Could you check a few things on this model? Use its own coordinates, in mm. Face numbers are marked on the shaded views. A direction names the side the tool comes from. Round coordinates to 2 decimals unless told otherwise and drop trailing zeros. Loops run counter-clockwise (first coordinate to the right, second up) from the corner with the lowest first, then second, coordinate; pieces in that order, holes last. Notation, with made-up numbers: (72.25, 84) -> (108.25, 84) arc R23 ccw to (108.25, 105) -> close; hole circle Ø10 at (64.25, 82). An arc over 180 degrees is marked (long way). One line per item, written item: value.
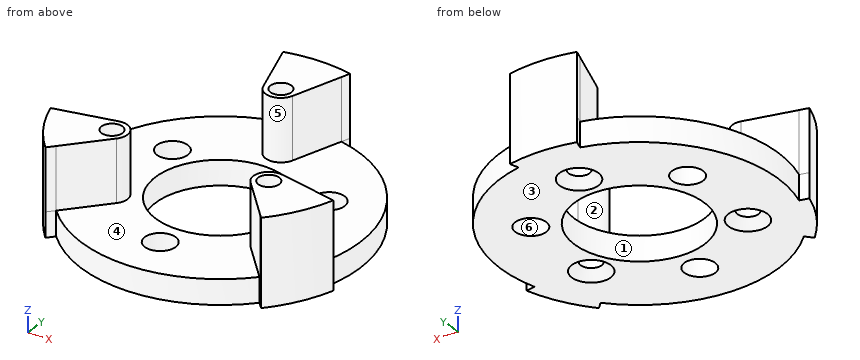
```python
from build123d import *

# Parameters (mm, degrees)
SKETCH1_R                                       = 22.5
SKETCH1_R_2                                     = 10.5
SKETCH1_R_3                                     = 1.5
BOSS_EXTRUDE1_DEPTH                             = 4
BOSS_EXTRUDE4_START                             = -4
SKETCH4_R                                       = 2.5
SKETCH4_R_2                                     = 1.5
BOSS_EXTRUDE4_DEPTH                             = 4
SKETCH4_5_R                                     = 1.5
BOSS_EXTRUDE5_DEPTH                             = 10
CUT_EXTRUDE1_DEPTH                              = 35.690393407
CUT_EXTRUDE1_DEPTH_BACK                         = 35.690393407
SKETCH4_3_R                                     = 2.5
CSK_FOR_M3_FLAT_HEAD_MACHINE_SCREW1_D           = 3.4
CSK_FOR_M3_FLAT_HEAD_MACHINE_SCREW1_CSINK_D     = 6.3
CSK_FOR_M3_FLAT_HEAD_MACHINE_SCREW1_CSINK_ANGLE = 90


with BuildPart() as part:
    # Sketch1 → Boss-Extrude1 (new body)
    with BuildSketch(Plane.XY):
        Circle(SKETCH1_R)
        Circle(SKETCH1_R_2, mode=Mode.SUBTRACT)
        with Locations((12.730573436, -7.35)):
            Circle(SKETCH1_R_3, mode=Mode.SUBTRACT)
        with Locations((0, 14.7)):
            Circle(SKETCH1_R_3, mode=Mode.SUBTRACT)
        with Locations((-12.730573436, -7.35)):
            Circle(SKETCH1_R_3, mode=Mode.SUBTRACT)
    extrude(amount=BOSS_EXTRUDE1_DEPTH)

    # Sketch4 → Boss-Extrude4 (add)
    # profile 1 of 6: a face of its own
    with BuildSketch(Plane.XY.offset(4).offset(BOSS_EXTRUDE4_START)):
        with Locations((0, -14.7)):
            Circle(SKETCH4_R)
    # profile 2 of 6: a face of its own
    with BuildSketch(Plane.XY.offset(4).offset(BOSS_EXTRUDE4_START)):
        with Locations((-12.730573436, 7.35)):
            Circle(SKETCH4_R)
    # profile 3 of 6: a face of its own
    with BuildSketch(Plane.XY.offset(4).offset(BOSS_EXTRUDE4_START)):
        with Locations((12.730573436, 7.35)):
            Circle(SKETCH4_R)
    # profile 4 of 6: a face of its own
    with BuildSketch(Plane.XY.offset(4).offset(BOSS_EXTRUDE4_START)):
        with BuildLine():
            Line((-10.872711372, -9.022826516), (-17.518780447, -16.404034005))
            ThreePointArc((-17.518780447, -16.404034005), (-20.784609691, -12), (-22.965700397, -6.969691908))
            Line((-22.965700397, -6.969691908), (-13.250352663, -4.904630998))
            ThreePointArc((-13.250352663, -4.904630998), (-10.565509926, -6.1), (-10.872711372, -9.022826516))
        make_face()
        with Locations((-12.730573436, -7.35)):
            Circle(SKETCH4_R_2, mode=Mode.SUBTRACT)
    # profile 5 of 6: a face of its own
    with BuildSketch(Plane.XY.offset(4).offset(BOSS_EXTRUDE4_START)):
        with BuildLine():
            Line((2.377641291, 13.927457514), (5.44691995, 23.373725913))
            ThreePointArc((5.44691995, 23.373725913), (0, 24), (-5.44691995, 23.373725913))
            Line((-5.44691995, 23.373725913), (-2.377641291, 13.927457514))
            ThreePointArc((-2.377641291, 13.927457514), (0, 12.2), (2.377641291, 13.927457514))
        make_face()
        with Locations((0, 14.7)):
            Circle(SKETCH4_R_2, mode=Mode.SUBTRACT)
    # profile 6 of 6: a face of its own
    with BuildSketch(Plane.XY.offset(4).offset(BOSS_EXTRUDE4_START)):
        with BuildLine():
            Line((10.872711372, -9.022826516), (17.518780447, -16.404034005))
            ThreePointArc((17.518780447, -16.404034005), (20.784609691, -12), (22.965700397, -6.969691908))
            Line((22.965700397, -6.969691908), (13.250352663, -4.904630998))
            ThreePointArc((13.250352663, -4.904630998), (10.565509926, -6.1), (10.872711372, -9.022826516))
        make_face()
        with Locations((12.730573436, -7.35)):
            Circle(SKETCH4_R_2, mode=Mode.SUBTRACT)
    extrude(amount=BOSS_EXTRUDE4_DEPTH)

    # Sketch4<5> → Boss-Extrude5 (add)
    # profile 1 of 6: a face of its own
    with BuildSketch(Plane.XY.offset(4)):
        with BuildLine():
            Line((-5.44691995, 23.373725913), (-4.981593415, 21.941598097))
            ThreePointArc((-4.981593415, 21.941598097), (0, 22.5), (4.981593415, 21.941598097))
            Line((4.981593415, 21.941598097), (5.44691995, 23.373725913))
            ThreePointArc((5.44691995, 23.373725913), (0, 24), (-5.44691995, 23.373725913))
        make_face()
    # profile 2 of 6: a face of its own
    with BuildSketch(Plane.XY.offset(4)):
        with BuildLine():
            ThreePointArc((4.981593415, 21.941598097), (0, 22.5), (-4.981593415, 21.941598097))
            Line((-4.981593415, 21.941598097), (-2.377641291, 13.927457514))
            ThreePointArc((-2.377641291, 13.927457514), (0, 12.2), (2.377641291, 13.927457514))
            Line((2.377641291, 13.927457514), (4.981593415, 21.941598097))
        make_face()
        with Locations((0, 14.7)):
            Circle(SKETCH4_5_R, mode=Mode.SUBTRACT)
    # profile 3 of 6: a face of its own
    with BuildSketch(Plane.XY.offset(4)):
        with BuildLine():
            Line((-17.518780447, -16.404034005), (-16.511184644, -15.284985497))
            ThreePointArc((-16.511184644, -15.284985497), (-19.485571585, -11.25), (-21.492778059, -6.6566126))
            Line((-21.492778059, -6.6566126), (-22.965700397, -6.969691908))
            ThreePointArc((-22.965700397, -6.969691908), (-20.784609691, -12), (-17.518780447, -16.404034005))
        make_face()
    # profile 4 of 6: a face of its own
    with BuildSketch(Plane.XY.offset(4)):
        with BuildLine():
            Line((-16.511184644, -15.284985497), (-10.872711372, -9.022826516))
            ThreePointArc((-10.872711372, -9.022826516), (-10.565509926, -6.1), (-13.250352663, -4.904630998))
            Line((-13.250352663, -4.904630998), (-21.492778059, -6.6566126))
            ThreePointArc((-21.492778059, -6.6566126), (-19.485571585, -11.25), (-16.511184644, -15.284985497))
        make_face()
        with Locations((-12.730573436, -7.35)):
            Circle(SKETCH4_5_R, mode=Mode.SUBTRACT)
    # profile 5 of 6: a face of its own
    with BuildSketch(Plane.XY.offset(4)):
        with BuildLine():
            Line((10.872711372, -9.022826516), (16.511184644, -15.284985497))
            ThreePointArc((16.511184644, -15.284985497), (19.485571585, -11.25), (21.492778059, -6.6566126))
            Line((21.492778059, -6.6566126), (13.250352663, -4.904630998))
            ThreePointArc((13.250352663, -4.904630998), (10.565509926, -6.1), (10.872711372, -9.022826516))
        make_face()
        with Locations((12.730573436, -7.35)):
            Circle(SKETCH4_5_R, mode=Mode.SUBTRACT)
    # profile 6 of 6: a face of its own
    with BuildSketch(Plane.XY.offset(4)):
        with BuildLine():
            ThreePointArc((21.492778059, -6.6566126), (19.485571585, -11.25), (16.511184644, -15.284985497))
            Line((16.511184644, -15.284985497), (17.518780447, -16.404034005))
            ThreePointArc((17.518780447, -16.404034005), (20.784609691, -12), (22.965700397, -6.969691908))
            Line((22.965700397, -6.969691908), (21.492778059, -6.6566126))
        make_face()
    extrude(amount=BOSS_EXTRUDE5_DEPTH)

    # Sketch4<3> → Cut-Extrude1 (cut, two sides: drawn at the far end of the back side and taken through both)
    with BuildSketch(Plane.XY.offset(4).offset(-CUT_EXTRUDE1_DEPTH_BACK)):
        with Locations((0, -14.7)):
            Circle(SKETCH4_3_R)
        with Locations((-12.730573436, 7.35)):
            Circle(SKETCH4_3_R)
        with Locations((12.730573436, 7.35)):
            Circle(SKETCH4_3_R)
    extrude(amount=CUT_EXTRUDE1_DEPTH + CUT_EXTRUDE1_DEPTH_BACK, mode=Mode.SUBTRACT)

    # CSK for M3 Flat Head Machine Screw1 (through all)
    with Locations(Plane(origin=(0, 0, 0), x_dir=(-1, 0, 0), z_dir=(0, 0, -1))):
        with Locations((12.730573436, -7.35), (0, 14.7), (-12.730573436, -7.35)):
            CounterSinkHole(CSK_FOR_M3_FLAT_HEAD_MACHINE_SCREW1_D / 2, CSK_FOR_M3_FLAT_HEAD_MACHINE_SCREW1_CSINK_D / 2, counter_sink_angle=CSK_FOR_M3_FLAT_HEAD_MACHINE_SCREW1_CSINK_ANGLE)


solid = part.part
```
(1) On a 3-axis mill with a long thin cutter (end or side, diameter ignored), from which of +Z, -Z, +X, -X, +Y, -Y can I reach the whole of each face in a straight line? I mean the marked faces 4, 5 and 6. Say none if no direction works.
Results below:
face 4: +Z
face 5: +Z, -Y
face 6: +Z, -Z
(2) Imagine slicing it at B-B on z = 12. Write out the boundary of the cut face in (x, y).
Results below:
outline: (-22.97, -6.97) arc R24 ccw to (-17.52, -16.4) -> (-10.87, -9.02) arc R2.5 ccw to (-13.25, -4.9) -> close; (-5.45, 23.37) -> (-2.38, 13.93) arc R2.5 ccw to (2.38, 13.93) -> (5.45, 23.37) arc R24 ccw to start; (10.87, -9.02) -> (17.52, -16.4) arc R24 ccw to (22.97, -6.97) -> (13.25, -4.9) arc R2.5 ccw to start; hole circle Ø3.4 at (-12.73, -7.35); hole circle Ø3.4 at (0, 14.7); hole circle Ø3.4 at (12.73, -7.35)
(3) We'd pull the mould along Y, two halves only. Please class the marked faces 1, 2 and 3: +Y half, -Y half, draft (parallel to the pull), parting line (faces both ways), or undercut.
Results below:
face 1: undercut
face 2: parting line
face 3: draft
(4) Imagine slicing it at A-A on x = 0. Write out the boundary of the cut face in (y, z), then the cut area to 3 significant figures.
Results below:
outline: (-22.5, 0) -> (-17.2, 0) -> (-17.2, 4) -> (-22.5, 4) -> close; (-12.2, 0) -> (-10.5, 0) -> (-10.5, 4) -> (-12.2, 4) -> close; (10.5, 0) -> (11.55, 0) -> (13, 1.45) -> (13, 14) -> (12.2, 14) -> (12.2, 4) -> (10.5, 4) -> close; (16.4, 1.45) -> (17.85, 0) -> (24, 0) -> (24, 14) -> (16.4, 14) -> close
area: 150 mm²
(5) Please list where these lines run through material, in increasing order: L1, parallel to Y at x = 0, z = 8.5; L2, parallel to Y at x = 0, z = 1.15; L3, parallel to X at y = 7.35, z = 1.7.
Results below:
L1: y = 12.2 to 13, 16.4 to 24
L2: y = -22.5 to -17.2, -12.2 to -10.5, 10.5 to 12.7, 16.7 to 24
L3: x = -21.27 to -15.23, -10.23 to -7.5, 7.5 to 10.23, 15.23 to 21.27
(6) Imagine slicing it at C-C on y = 0. Write out the boundary of the cut face in (x, z), then the cut area to 3 significant figures.
Results below:
outline: (-22.5, 0) -> (-10.5, 0) -> (-10.5, 4) -> (-22.5, 4) -> close; (10.5, 0) -> (22.5, 0) -> (22.5, 4) -> (10.5, 4) -> close
area: 96.0 mm²
(7) For pin 1 Ø10 at (x, y) = (0.5, -2) entering from -Z; pin 2 Ø4 at (x, y) = (0, 14.7) entering from -Z; pin 3 Ø1.5 at (y, z) = (-8, 11.5) entering from +X; pin 4 Ø6 at (x, y) = (16, 0) entering from +Z, each with a flat end and sliding along its axis, tell me the tip position at first contact or that it passes through.
Results below:
pin 1: passes through
pin 2: stops at z = 1.15
pin 3: stops at x = 22.88
pin 4: stops at z = 4
(8) Imagine slicing it at D-D on x = 6. Write out the boundary of the cut face in (y, z), then the cut area to 3 significant figures.
Results below:
outline: (-21.69, 0) -> (-8.62, 0) -> (-8.62, 4) -> (-21.69, 4) -> close; (8.62, 0) -> (21.69, 0) -> (21.69, 4) -> (8.62, 4) -> close
area: 105 mm²
